```python
from build123d import *

# Parameters (mm, degrees)
F0_W     = 152.4
F0_H     = 82.55
F1_DEPTH = 25.4
F3_DEPTH = 25.4
F4_R     = 3.175
F5_DEPTH = 25.4
F6_SIZE  = 6.35


with BuildPart() as f1:
    # F0 (on Top) → F1 (new body)
    with BuildSketch(Plane.XY):
        Rectangle(F0_W, F0_H)
    extrude(amount=F1_DEPTH)

    # F2 (on Front) → F3 (join)
    with BuildSketch(Plane.XZ):
        Polygon((63.5, 0), (0, 0), (-63.5, 0), (-63.5, -25.4), (63.5, -25.4), align=None)
    extrude(amount=F3_DEPTH)

    # F4 (on face) → F5 (cut)
    with BuildSketch(Plane.XZ.offset(25.4)):
        with BuildLine():
            Line((3.175, -12.7), (0, -12.7))
            Line((0, -12.7), (-3.175, -12.7))
            ThreePointArc((-3.175, -12.7), (0, -15.875), (3.175, -12.7))
        make_face()
        with BuildLine():
            Line((-3.175, -12.7), (0, -12.7))
            Line((0, -12.7), (3.175, -12.7))
            ThreePointArc((3.175, -12.7), (0, -9.525), (-3.175, -12.7))
        make_face()
        with Locations((-50.8, -12.7)):
            Circle(F4_R)
        with BuildLine():
            ThreePointArc((53.975, -12.7), (50.8, -9.525), (47.625, -12.7))
            ThreePointArc((47.625, -12.7), (50.8, -15.875), (53.975, -12.7))
        make_face()
    extrude(amount=-F5_DEPTH, mode=Mode.SUBTRACT)

    # F6
    f6_edges = [f1.edges().sort_by_distance(p)[0] for p in [
        (0, 41.275, 25.4),
        (-76.2, 0, 25.4),
        (0, -41.275, 25.4),
        (76.2, 0, 25.4),
    ]]
    chamfer(f6_edges, length=F6_SIZE)


solid = f1.part
```
Source: CAD feature listing. Evaluate the final solid. Frame: model axes, mm. A direction names the side the tool comes from. Round coordinates to 2 decimals unless told otherwise and drop trailing zeros. Loops run counter-clockwise (first coordinate to the right, second up) from the corner with the lowest first, then second, coordinate; pieces in that order, holes last. Notation, with made-up numbers: M 47.25,-14.75 L 93.25,-14.75 A11 ccw 93.25,3.25 Z; hole C -2.75,-8 d1. An arc over 180 degrees is marked long. Use a Markdown table: item, result. Add a question column.
1. Section query C-C on y = -3. Return the cut outline in (x, z) (3 decimals), then the cut area to 3 significant figures.
2. Section query D-D on x = 57.5. Return the cut outline in (y, z) (3 decimals), then the cut area to 3 significant figures.
3. Line query: line 1 (X direction, y = -6, z = -12); line 2 (Z direction, x = -50.8, y = -10.25) (3 decimals); line 3 (Y direction, x = -7, z = -4). Output: solid intervals per line, ascending.
4. Section query A-A on x = -50.8. Return the cut outline in (y, z) (3 decimals).
5. Reachability of faces 1 (the flat face through (-63.5, -13, -13)), 2 (the flat face through (-1, -25.4, -18)), 3 (the flat face through (-1, -41.275, 9)) from +Z, -Z, +X, -X, +Y, -Y: full face, straight path, thin tool, end or side. Return the list, or none.
6. Mould query, pull axis X, two halves, no side actions, for faces 4 (the flat face through (-72.98, -0.58, 22.27)), 5 (the flat face through (63.5, -13, -13)), 6 (the flat face through (-1, 0, -18)), 7 (the cylindrical face through (53.97, -12.88, -12.84)). Classes: pulls with the +X half, pulls with the -X half, needs draft (parallel to the pull), parting line crosses it, or undercut.
7. Section query B-B on z = -12.7. Return the cut outline in (x, y) (3 decimals).
8. Contact query for flat-ended pins moving along their axis: P1, Ø10, axis at x = 33, z = -14.5, coming from the -Y side; P2, Ø1.5, axis at x = -57.5, z = -13.5, coming from the +Y side; P3, Ø7.5, axis at y = -16, z = -6.5, coming from the -X side. Output: stop coordinate, or through.
Reported:
| question | item | result |
|---|---|---|
| 1 | outline | M -76.2,0 L -63.5,0 L -63.5,-25.4 L 63.5,-25.4 L 63.5,0 L 76.2,0 L 76.2,19.05 L 69.85,25.4 L -69.85,25.4 L -76.2,19.05 Z; hole C -50.8,-12.7 d6.35; hole C 0,-12.7 d6.35; hole C 50.8,-12.7 d6.35 |
| 1 | area | 6,960 mm² |
| 2 | outline | M -41.275,0 L -25.4,0 L -25.4,-25.4 L 0,-25.4 L 0,0 L 41.275,0 L 41.275,19.05 L 34.925,25.4 L -34.925,25.4 L -41.275,19.05 Z |
| 2 | area | 2,700 mm² |
| 3 | line 1 | x = -63.5 to -53.9, -47.7 to -3.1, 3.1 to 47.7, 53.9 to 63.5 |
| 3 | line 2 | z = -25.4 to -15.875, -9.525 to 25.4 |
| 3 | line 3 | y = -25.4 to 0 |
| 4 | outline | M -41.275,0 L -25.4,0 L -25.4,-9.525 L 0,-9.525 L 0,0 L 41.275,0 L 41.275,19.05 L 34.925,25.4 L -34.925,25.4 L -41.275,19.05 Z; M -25.4,-25.4 L 0,-25.4 L 0,-15.875 L -25.4,-15.875 Z |
| 5 | face 1 | -Z, -X, +Y, -Y |
| 5 | face 2 | -Z, +X, -X, -Y |
| 5 | face 3 | +Z, -Z, +X, -X, -Y |
| 6 | face 4 | pulls with the -X half |
| 6 | face 5 | pulls with the +X half |
| 6 | face 6 | needs draft |
| 6 | face 7 | undercut |
| 7 | outline | M -63.5,-25.4 L -53.975,-25.4 L -53.975,0 L -63.5,0 Z; M -47.625,-25.4 L -3.175,-25.4 L -3.175,0 L -47.625,0 Z; M 3.175,-25.4 L 47.625,-25.4 L 47.625,0 L 3.175,0 Z; M 53.975,-25.4 L 63.5,-25.4 L 63.5,0 L 53.975,0 Z |
| 8 | P1 | stops at y = -25.4 |
| 8 | P2 | stops at y = 0 |
| 8 | P3 | stops at x = -63.5 |
